from build123d import *

# Parameters (mm, degrees)
SKETCH1_R               = 21
BOSS_EXTRUDE1_DEPTH     = 5
SKETCH2_R               = 4.863
BOSS_EXTRUDE2_DEPTH     = 7
SWEEP1_PITCH            = 1.75
CUT_EXTRUDE1_DEPTH      = 33.325986764
CUT_EXTRUDE1_DEPTH_BACK = 33.325986764


with BuildPart() as part:
    # Sketch1 → Boss-Extrude1 (new body)
    with BuildSketch(Plane(origin=(0, 0, 0), x_dir=(1, 0, 0), z_dir=(0, 1, 0))):
        with Locations(Location((0, 0, 0), (0, 0, 270))):
            Circle(SKETCH1_R)
    extrude(amount=-BOSS_EXTRUDE1_DEPTH)

    # Sketch2 → Boss-Extrude2 (add)
    with BuildSketch(Plane.XZ.offset(5)):
        with Locations(Location((0, 0, 0), (0, 0, 90))):
            Circle(SKETCH2_R)
    extrude(amount=BOSS_EXTRUDE2_DEPTH)

    # Sweep1: arcs per turn and ends read off the stored shape
    # Sweep1: the profile of Sketch11 screwed along a left-hand helix through 4 turns, 10 arcs to a turn; built about Z, then put on its axis
    sweep1_z = Axis((0, 0, 0), (0, 0, 1))
    sweep1_corners = [(4.826232454, 0, 0), (4.826232454, 0, -0.765947256), (5.963232454, 0, -0.1095), (5.963232454, 0, 0.1095), (4.826232454, 0, 0.765947256)]
    with BuildLine(mode=Mode.PRIVATE) as sweep1_profile:
        Line(sweep1_corners[0], sweep1_corners[1])
        Line(sweep1_corners[1], sweep1_corners[2])
        Line(sweep1_corners[2], sweep1_corners[3])
        Line(sweep1_corners[3], sweep1_corners[4])
        Line(sweep1_corners[4], sweep1_corners[0])
    sweep1_cap = Face(sweep1_profile.wire())
    sweep1_turn_angles = [0, -18, -36, -54, -72, -90, -108, -126, -144, -162, -180, -198, -216, -234, -252, -270, -288, -306, -324, -342, -360]
    sweep1_turn_weights = [1, 0.9510565162951535, 1, 0.9510565162951535, 1, 0.9510565162951535, 1, 0.9510565162951535, 1, 0.9510565162951535, 1, 0.9510565162951535, 1, 0.9510565162951535, 1, 0.9510565162951535, 1, 0.9510565162951535, 1, 0.9510565162951535, 1]
    sweep1_turn_rails = [Edge.make_bspline([Vector(p[0], p[1], 0).rotate(sweep1_z, sweep1_turn_angles[k]) / sweep1_turn_weights[k] + Vector(0, 0, p[2] + -SWEEP1_PITCH * sweep1_turn_angles[k] / 360) for k in range(21)], [0, 0, 0, 1, 1, 2, 2, 3, 3, 4, 4, 5, 5, 6, 6, 7, 7, 8, 8, 9, 9, 10, 10, 10], 2, sweep1_turn_weights) for p in sweep1_corners]
    sweep1_turn_sides = [Face.make_surface_from_curves(sweep1_turn_rails[p[0]], sweep1_turn_rails[p[1]]) for p in [(0, 1), (1, 2), (2, 3), (3, 4), (4, 0)]]
    sweep1 = Plane(origin=(0, -12, 0), x_dir=(1, 0, 0), z_dir=(0, 1, 0)) * Solid(Shell([*[p.moved(Location((0, 0, SWEEP1_PITCH * i))) for i in range(4) for p in sweep1_turn_sides], sweep1_cap, sweep1_cap.rotate(sweep1_z, -1440).moved(Location((0, 0, -SWEEP1_PITCH * -1440 / 360)))]))
    add(sweep1)

    # Sketch12 → Cut-Extrude1 (cut, two sides: drawn at the far end of the back side and taken through both)
    with BuildSketch(Plane.XY.offset(-CUT_EXTRUDE1_DEPTH_BACK)):
        Polygon((0, -12), (5.963232454, -12), (5.963232454, -12.765947256), (0, -12.765947256), (-4.863, -12.765947256), (-4.863, -12), align=None)
    extrude(amount=CUT_EXTRUDE1_DEPTH + CUT_EXTRUDE1_DEPTH_BACK, mode=Mode.SUBTRACT)


solid = part.part
Geometry: final body of the model. Coordinates: model frame, mm. Give positions to 0.01 mm unless a question says otherwise; leave off trailing zeros. Loops run counter-clockwise (first coordinate to the right, second up) from the corner with the lowest first, then second, coordinate; pieces in that order, holes last. Notation, with made-up numbers: (-38, 87) - (-9, 87) arc R29 ccw to (-9, 121) - close; hole circle Ø1 at (67.5, 16.25). An arc over 180 degrees is marked (long way). One line per question, with ' | ' between items. Start each with the question number.
(1) Section query A-A on x = 16. Return loops of the section in (y, z), then the cut area to 3 significant figures.
(2) Ray query, line 1 (Y direction, x = 0, z = -5); line 2 (Y direction, x = 17, z = 5.5); line 3 (Z direction, x = -15.5, y = -2). Return the intervals inside material, ascending. Write a range as from..to.
(3) Section query B-B on z = -11. Return loops of the section in (x, y).
(4) Contact query for flat-ended pins moving along their axis: pin 1 (0.8 mm diameter, centred on x = 5.5, y = -11.5, fed in from -Z); pin 2 (1.5 mm diameter, centred on y = -7.5, z = -2, fed in from +X); pin 3 (21 mm diameter, centred on x = 9.5, z = 1, fed in from -Y); pin 4 (2 mm diameter, centred on y = -3.5, z = -2, fed in from -X). Output: stop coordinate, or through.
The answers:
1) outline: (-5, -13.6) - (0, -13.6) - (0, 13.6) - (-5, 13.6) - close | area: 136 mm2
2) line 1: -11.35..-10.02, -9.6..-8.27, -7.85..-6.52, -6.1..0 | line 2: -5..0 | line 3: -14.17..14.17
3) outline: (-17.89, -5) - (17.89, -5) - (17.89, 0) - (-17.89, 0) - close
4) pin 1: z = 0 | pin 2: x = 5.77 | pin 3: y = -12 | pin 4: x = -20.98
